Geometry check sheet. Reference: the model listing, model coordinates, mm. A direction names the side the tool comes from. Give positions to 0.01 mm unless a question says otherwise; leave off trailing zeros. Write each loop counter-clockwise with the first axis right and the second up, starting at its lowest first coordinate (ties: lowest second). Pieces come first, ordered by that corner, then holes.
(1) Mould release check, pull along Y, two halves, no side actions. Record for faces 1 (the flat face through (0, 0, 180)), 2 (the cylindrical face through (-1.08, 4.88, 89.48)), 3 (the cylindrical face through (0.14, -4.88, -8.82)): +Y half, -Y half, draft (parallel to the pull), parting line (faces both ways), or undercut.
(2) Thickness scan on line 1 along Z through (x, y) = (-7, -0.25); line 2 along Z through (x, y) = (2, -0.5); line 3 along X through (y, z) = (0.25, 118.5). Record the ranges inside material, lowest first.
(3) Tool access check on faces 4 (the flat face through (-7.146, -7, 0)), 5 (the flat face through (7.146, -7, 0)), 6 (the flat face through (-5, 2, 1.468)). Record the directions out of +Z, -Z, +X, -X, +Y, -Y that give a thin tool (end or side, any length) a straight path to the whole face; none if there is none.
(4) Depth check by flat-ended pin: P1, Ø5, axis at y = 5.5, z = 23.5, coming from the -X side; P2, Ø4, axis at y = 3.5, z = 130.5, coming from the +X side; P3, Ø6, axis at y = 0, z = -9.9, coming from the +X side; P4, Ø10, axis at y = -0.5, z = 133, coming from the -X side. Enter the tip coordinate at first touch or a pass-through.
(5) Cross-section at B-B (z = 70). Record the boundary of the cut face in (x, y), and give its area (3 significant figures).
(6) Cross-section at A-A (x = 0). Record the boundary of the cut face in (y, z).
Autodesk Inventor part; units mm, degrees
ref_plane "Work Plane1" through (0, 0, 1.4685) normal (0, 0, 1) x (1, 0, 0)
ref_plane "YZ Plane" through (0, 0, 0) normal (1, 0, 0) x (0, 1, 0)
ref_plane "XZ Plane" through (0, 0, 0) normal (0, 1, 0) x (-1, 0, 0)
sketch "Sketch1" plane through (0, 0, 0) normal (0, 0, 1) x (1, 0, 0)
  circle A0 centre (0, 0) radius 5
  dimension "d0" = 10
extrude "Extrusion1" add sketch "Sketch1" along normal blind 180
thread "Thread1"
sketch "Sketch2" plane through (0, 0, 0) normal (1, 0, 0) x (0, 1, 0)
  circle A0 centre (0, -9.9047) radius 11.3732
  point P0 (0, 0)
extrude "Extrusion2" add sketch "Sketch2" along normal mid plane 20
sketch "Sketch3" plane through (10, 0, -9.9047) normal (1, 0, 0) x (0, 0, -1)
  circle A0 centre (0, 0) radius 5
  point P0 (-9.9047, 0)
  dimension "d7" = 10
extrude "Extrusion3" cut sketch "Sketch3" against normal blind 20
fillet "Fillet1" radius 2 2 edges at (10, -11.3732, -9.9047) (-10, -11.3732, -9.9047)
ref_plane "Work Plane1" through (0, 0, 1.4685) normal (0, 0, 1) x (1, 0, 0)
sketch "Sketch4" plane through (0, 0, 1.4685) normal (0, 0, 1) x (1, 0, 0)
  line L0 (-7.1456, 9.3732) -> (7.1456, 9.3732)
  line L1 (7.1456, 9.3732) -> (7.1456, -9.3732)
  line L2 (7.1456, -9.3732) -> (-7.1456, -9.3732)
  line L3 (-7.1456, -9.3732) -> (-7.1456, 9.3732)
  line L4 (-7.1456, 9.3732) -> (7.1456, -9.3732) construction
  line L5 (7.1456, 9.3732) -> (-7.1456, -9.3732) construction
  point P0 (0, 0)
extrude "Extrusion4" add sketch "Sketch4" against normal blind 5
fillet "Fillet2" radius 2 2 edges at (0, 9.3732, 1.4685) (0, -9.3732, 1.4685)
properties part number "rod"
Reply:
1. face 1: draft
1. face 2: parting line
1. face 3: undercut
2. line 1: z = -21.28 to -14.9, -4.91 to 1.47
2. line 2: z = -21.27 to -14.88, -4.93 to 180
2. line 3: x = -4.99 to 4.99
3. face 4: +Z, -X, -Y
3. face 5: +Z, +X, -Y
3. face 6: +Z
4. P1: stops at x = -4
4. P2: stops at x = 4.77
4. P3: passes through
4. P4: stops at x = -5
5. outline: circle Ø10 at (0, 0)
5. area: 78.5 mm2
6. outline: (-9.37, -3.46) arc R11.37 ccw (long way) to (9.37, -3.46) - (9.37, -0.53) arc R2 ccw to (7.37, 1.47) - (5, 1.47) - (5, 180) - (-5, 180) - (-5, 1.47) - (-7.37, 1.47) arc R2 ccw to (-9.37, -0.53) - close; hole circle Ø10 at (0, -9.9)
